Drawing for the job (mm, zero at the part's lowest x, y, z). A direction names the side the tool comes from. Give positions to 0.01 mm unless a question says otherwise; leave off trailing zeros. Write each loop counter-clockwise with the first axis right and the second up, starting at its lowest first coordinate (ties: lowest second). Pieces come first, ordered by that corner, then holes.
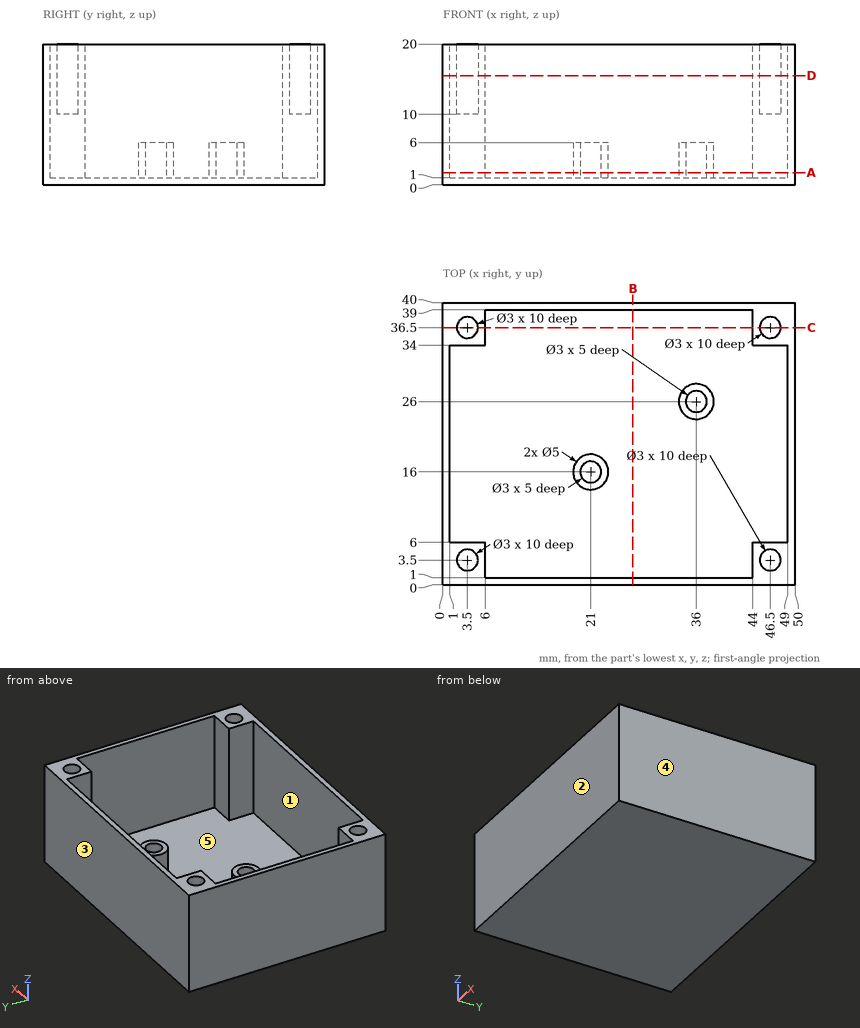
1. Pin check, flat tips, straight feed: P1, Ø1.5, axis at x = 3.5, y = 36.5, coming from the +Z side; P2, Ø2.5, axis at x = 20.5, y = 15.5, coming from the +Z side. Stop position of each tip, or through.
Calculated:
P1: stops at z = 10
P2: stops at z = 6
2. Pull direction X, two halves, no side cores. Call the marked faces 3, 4 and 5: +X half, -X half, draft (parallel to the pull), parting line (faces both ways), or undercut.
Calculated:
face 3: draft
face 4: +X half
face 5: undercut
3. Slice it at A-A, the plane z = 1.75. Write the cut outline in (x, y), and give its area (3 significant figures).
Calculated:
outline: (0, 0) - (50, 0) - (50, 40) - (0, 40) - close; circle Ø5 at (21, 16); circle Ø5 at (36, 26); hole (1, 6) - (6, 6) - (6, 1) - (44, 1) - (44, 6) - (49, 6) - (49, 34) - (44, 34) - (44, 39) - (6, 39) - (6, 34) - (1, 34) - close; hole circle Ø3 at (21, 16); hole circle Ø3 at (36, 26)
area: 301 mm2
4. Which spindle directions (+Z, -Z, +X, -X, +Y, -Y) get a long thin tool onto all of the face, cutting with end or side? Do the marked faces 1 and 2. Say none if no direction does.
Calculated:
face 1: +Z
face 2: +Z, -Z, +X, -X, -Y
5. Slice it at B-B, the plane x = 27. Write the cut outline in (y, z).
Calculated:
outline: (0, 0) - (40, 0) - (40, 20) - (39, 20) - (39, 1) - (1, 1) - (1, 20) - (0, 20) - close
6. Slice it at D-D, the plane z = 15.5. Write the cut outline in (x, y), and give its area (3 significant figures).
Calculated:
outline: (0, 0) - (50, 0) - (50, 40) - (0, 40) - close; hole (1, 6) - (6, 6) - (6, 1) - (44, 1) - (44, 6) - (49, 6) - (49, 34) - (44, 34) - (44, 39) - (6, 39) - (6, 34) - (1, 34) - close; hole circle Ø3 at (3.5, 3.5); hole circle Ø3 at (3.5, 36.5); hole circle Ø3 at (46.5, 3.5); hole circle Ø3 at (46.5, 36.5)
area: 248 mm2
7. Probe probe 1 along X at (y, z) = (3.5, 17.25); probe 2 along Y at (x, z) = (3.5, 12.75); probe 3 along Y at (x, z) = (45, 9.25). List the from-to ranges inside material, lowest first.
Calculated:
probe 1: x = 0 to 2, 5 to 6, 44 to 45, 48 to 50
probe 2: y = 0 to 2, 5 to 6, 34 to 35, 38 to 40
probe 3: y = 0 to 6, 34 to 40
8. Slice it at C-C, the plane y = 36.5. Write the cut outline in (x, z), and give its area (3 significant figures).
Calculated:
outline: (0, 0) - (50, 0) - (50, 20) - (48, 20) - (48, 10) - (45, 10) - (45, 20) - (44, 20) - (44, 1) - (6, 1) - (6, 20) - (5, 20) - (5, 10) - (2, 10) - (2, 20) - (0, 20) - close
area: 218 mm2
